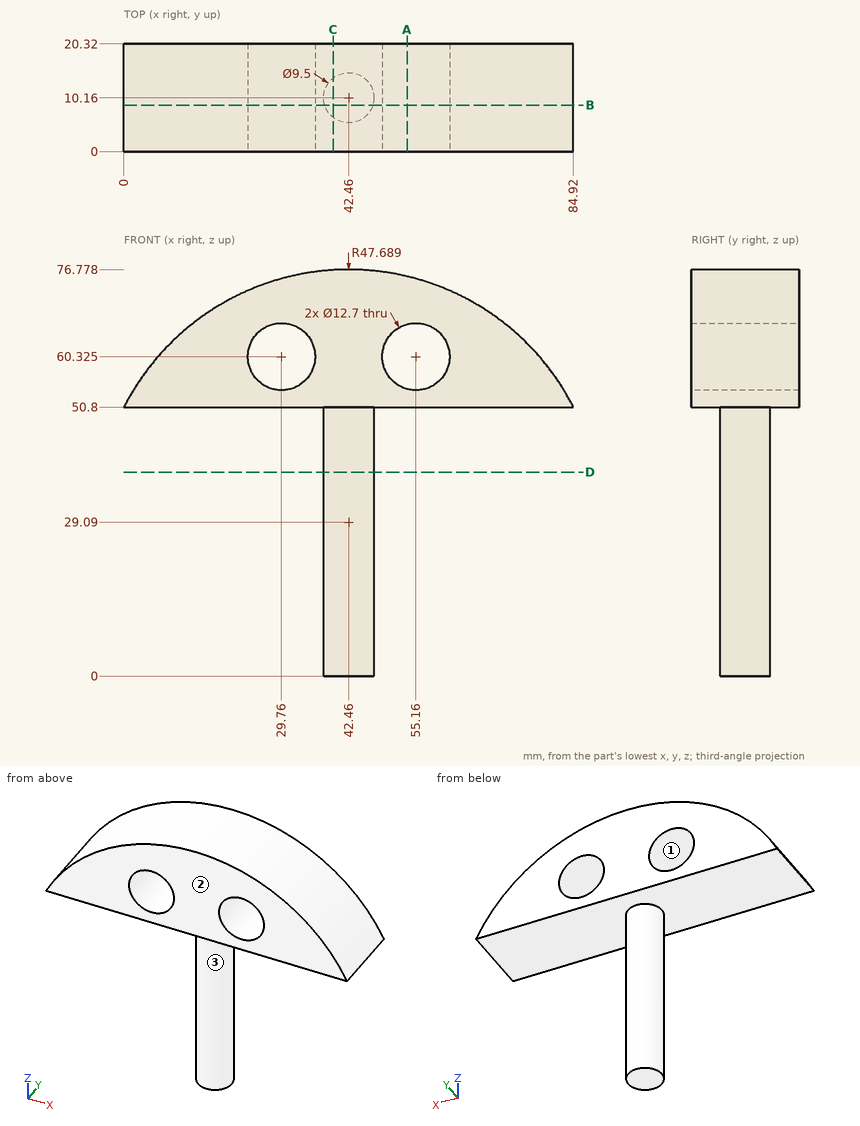
Could you check a few things on this drawing? It's one solid part, dimensions in mm from its lowest x, y, z. Give positions to 0.01 mm unless a question says otherwise; leave off trailing zeros. Write each loop counter-clockwise with the first axis right and the second up, starting at its lowest first coordinate (ties: lowest second). Pieces come first, ordered by that corner, then holes. Notation, with made-up numbers: (32, -35) - (43, -35) arc R29 ccw to (43, -13) - close; hole circle Ø8 at (-33.5, 79.25). An arc over 180 degrees is marked (long way). Use CSV: the item, a comma, the result in double quotes. Start each with the question number.
Item 1: If I drill on line 1 along Z through (x, y) = (33, 13.75) (1 decimal); line 2 along Z through (x, y) = (32.5, 11.25) (1 decimal); line 3 along Z through (x, y) = (11.5, 13.5), over which ranges is the centre line in solid material (lowest first)?
Item 2: If we mould it in two halves opening along X, with no side actions, what happens to the marked faces 1, 2 and 3? For each: pulls with the +X half, pulls with the -X half, needs draft (parallel to the pull), parting line crosses it, or undercut.
Item 3: I want a section at C-C, the plane x = 39.5. Please give me the cut outline in (y, z) (1 decimal).
Item 4: I'm going to push flat-ended pins straight in: pin 1 (12 mm diameter, centred on y = 8.5, z = 31.5, fed in from +X); pin 2 (3 mm diameter, centred on x = 56, y = 13, fed in from +Z); pin 3 (12 mm diameter, centred on y = 5, z = 44.5, fed in from -X); pin 4 (7.5 mm diameter, centred on x = 55.16, z = 60.32, fed in from -Y). Where does each tip first touch, or does it pass through?
Item 5: I want a section at D-D, the plane z = 38.5. Please give me the cut outline in (x, y).
Item 6: I want a section at B-B, the plane y = 8.75. Give the number of separate pieces and of enclosed holes in the cut face, then the cut area to 3 significant figures.
Item 7: I want a section at A-A, the plane x = 53.5. Please give me the cut outline in (y, z) (1 decimal).
Findings:
1,line 1,"z = 50.8 to 54.9, 65.8 to 75.8"
1,line 2,"z = 50.8 to 54.6, 66.1 to 75.7"
1,line 3,"z = 50.8 to 65.36"
2,face 1,"undercut"
2,face 2,"needs draft"
2,face 3,"parting line crosses it"
3,outline,"(0, 50.8) - (6.4, 50.8) - (6.4, 0) - (13.9, 0) - (13.9, 50.8) - (20.3, 50.8) - (20.3, 76.7) - (0, 76.7) - close"
4,pin 1,"stops at x = 47.21"
4,pin 2,"stops at z = 75.23"
4,pin 3,"stops at x = 37.71"
4,pin 4,"passes through"
5,outline,"circle Ø9.5 at (42.46, 10.16)"
6,separate pieces,"1"
6,enclosed holes,"2"
6,area,"1,780 mm2"
7,outline,"(0, 50.8) - (20.3, 50.8) - (20.3, 54.2) - (0, 54.2) - close; (0, 66.5) - (20.3, 66.5) - (20.3, 75.5) - (0, 75.5) - close"
